Here's how the part is built. I have some questions about the finished solid (model axes, mm). A direction names the side the tool comes from. Round coordinates to 2 decimals unless told otherwise and drop trailing zeros. Loops run counter-clockwise (first coordinate to the right, second up) from the corner with the lowest first, then second, coordinate; pieces in that order, holes last. Notation, with made-up numbers: M -11.75,53 L 7.25,53 A22 cw 7.25,91 Z; hole C 84.25,-22.75 d11. An arc over 180 degrees is marked long. Use a Markdown table: item, result.
```python
from build123d import *

# Parameters (mm, degrees)
PAD_DEPTH       = 18
SKETCH007_W     = 12.8
SKETCH007_H     = 45
POCKET002_DEPTH = 5
SKETCH010_W     = 27
SKETCH010_H     = 13
POCKET005_DEPTH = 5


with BuildPart() as part:
    # Clone2D → Pad (new body)
    with BuildSketch(Plane.YZ):
        with BuildLine():
            ThreePointArc((75, 196), (83.780456, 193.01205), (93, 192))
            Line((93, 192), (95, 192))
            Line((95, 192), (95, 0))
            Line((95, 0), (93, 0))
            ThreePointArc((93, 0), (83.780456, 1.01205), (75, 4))
            ThreePointArc((75, 4), (66.219544, 6.98795), (57, 8))
            Line((57, 8), (6.4, 8))
            Line((6.4, 8), (6.4, 17))
            Line((6.4, 17), (-6.4, 17))
            Line((-6.4, 17), (-6.4, 26))
            Line((-6.4, 26), (6.4, 26))
            Line((6.4, 26), (6.4, 35))
            Line((6.4, 35), (68, 35))
            Line((68, 35), (68, 48))
            Line((68, 48), (-6.4, 48))
            Line((-6.4, 48), (-6.4, 57))
            Line((-6.4, 57), (6.4, 57))
            Line((6.4, 57), (6.4, 66))
            Line((6.4, 66), (-6.4, 66))
            Line((-6.4, 66), (-6.4, 75))
            Line((-6.4, 75), (43.180653, 75))
            ThreePointArc((43.180653, 75), (56.219058, 77.049413), (68, 83))
            Line((68, 83), (68, 111))
            ThreePointArc((68, 111), (56.219058, 116.950587), (43.180653, 119))
            Line((43.180653, 119), (6.4, 119))
            Line((6.4, 119), (6.4, 137))
            Line((6.4, 137), (-6.4, 137))
            Line((-6.4, 137), (-6.4, 146))
            Line((-6.4, 146), (6.4, 146))
            Line((6.4, 146), (6.4, 173))
            Line((6.4, 173), (-6.4, 173))
            Line((-6.4, 173), (-6.4, 182))
            Line((-6.4, 182), (6.4, 182))
            Line((6.4, 182), (6.4, 200))
            Line((6.4, 200), (57, 200))
            ThreePointArc((57, 200), (66.219544, 198.98795), (75, 196))
        make_face()
    extrude(amount=PAD_DEPTH)

    # Sketch007 (on Face38 of Pad) → Pocket002 (cut)
    with BuildSketch(Plane.YZ.offset(18)):
        with Locations((0, 159.5)):
            Rectangle(SKETCH007_W, SKETCH007_H)
    extrude(amount=-POCKET002_DEPTH, mode=Mode.SUBTRACT)

    # Sketch010 (on Face5 of Pocket002) → Pocket005 (cut)
    with BuildSketch(Plane.YZ.offset(18)):
        with Locations((81.5, 41.5)):
            Rectangle(SKETCH010_W, SKETCH010_H)
    extrude(amount=-POCKET005_DEPTH, mode=Mode.SUBTRACT)


solid = part.part
```
Q1. For faces 4 (the flat face through (9, 0, 17)), 5 (the flat face through (6, 0, 137)), 6 (the flat face through (9, -6.4, 52)), 7 (the flat face through (6, 0, 182)), 8 (the flat face through (13, 81, 42)), which set-ups out of +Z, -Z, +X, -X, +Y, -Y let a thin tool reach every point of the face, with its end or its side?
Return value:
| item | result |
|---|---|
| face 4 | -Z, +X, -X, -Y |
| face 5 | +X, -X, -Y |
| face 6 | +Z, -Z, +X, -X, -Y |
| face 7 | +Z, +X, -X, -Y |
| face 8 | +X, +Y, -Y |
Q2. Will these pins go through, and if not, where does the flat tip stop? P1, Ø1.6, axis at x = 8, y = 94, coming from the +Z side; P2, Ø6.5, axis at x = 7, y = -2, coming from the -Z side; P3, Ø4, axis at x = 8, y = 2, coming from the +Z side.
Return value:
| item | result |
|---|---|
| P1 | stops at z = 192 |
| P2 | stops at z = 17 |
| P3 | stops at z = 182 |
Q3. Imagine slicing it at A-A, the plane y = 4. Please give me the cut outline in (x, z).
Return value:
| item | result |
|---|---|
| outline | M 0,17 L 18,17 L 18,26 L 0,26 Z; M 0,48 L 18,48 L 18,57 L 0,57 Z; M 0,66 L 18,66 L 18,75 L 0,75 Z; M 0,137 L 13,137 L 13,146 L 0,146 Z; M 0,173 L 13,173 L 13,182 L 0,182 Z |
Q4. Imagine slicing it at D-D, the plane z = 157.5. Please give me the cut outline in (x, y), then the cut area to 3 significant figures.
Return value:
| item | result |
|---|---|
| outline | M 0,6.4 L 18,6.4 L 18,95 L 0,95 Z |
| area | 1,590 mm^2 |
Q5. Imagine slicing it at C-C, the plane y = 38.5. Please give me the cut outline in (x, z), then the cut area to 3 significant figures.
Return value:
| item | result |
|---|---|
| outline | M 0,8 L 18,8 L 18,35 L 0,35 Z; M 0,48 L 18,48 L 18,75 L 0,75 Z; M 0,119 L 18,119 L 18,200 L 0,200 Z |
| area | 2,430 mm^2 |
Q6. We'd pull the mould along Z, two halves only. Please class faces 1 (the flat face through (9, 6.4, 30)), 2 (the flat face through (13, 0, 178)), 3 (the flat face through (9, 31, 200)): pulls with the +Z half, pulls with the -Z half, needs draft (parallel to the pull), parting line crosses it, or undercut.
Return value:
| item | result |
|---|---|
| face 1 | undercut |
| face 2 | needs draft |
| face 3 | pulls with the +Z half |
Q7. I need wall thicknesses on line 1 (Z direction, x = 4, y = 39.5); line 2 (Z direction, x = 10.25, y = 56); line 3 (Y direction, x = 3.75, z = 132). Which ranges of each line are inside material? Lowest first, please. Write a range as from..to.
Return value:
| item | result |
|---|---|
| line 1 | z = 8..35, 48..75, 119..200 |
| line 2 | z = 8..35, 48..76.98, 117.02..200 |
| line 3 | y = 6.4..95 |
Q8. Imagine slicing it at B-B, the plane x = 15.75. Please give me the cut outline in (y, z).
Return value:
| item | result |
|---|---|
| outline | M -6.4,17 L 6.4,17 L 6.4,8 L 57,8 A42.5 cw 75,4 A42.5 ccw 93,0 L 95,0 L 95,35 L 6.4,35 L 6.4,26 L -6.4,26 Z; M -6.4,48 L 95,48 L 95,192 L 93,192 A42.5 cw 75,196 A42.5 ccw 57,200 L 6.4,200 L 6.4,119 L 43.18,119 A42.5 cw 68,111 L 68,83 A42.5 cw 43.18,75 L -6.4,75 L -6.4,66 L 6.4,66 L 6.4,57 L -6.4,57 Z |
